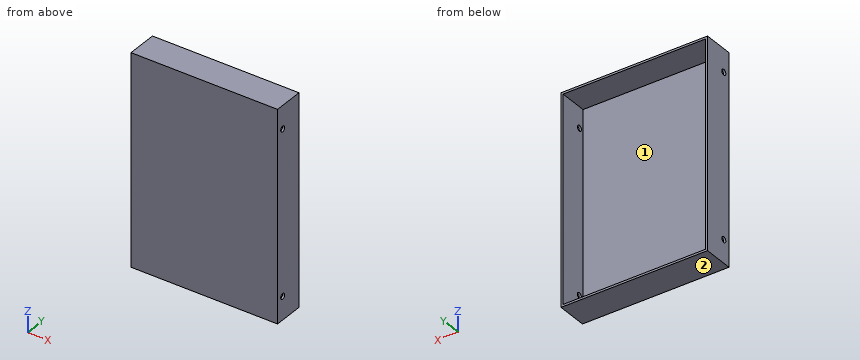
```python
from build123d import *

# Parameters (mm, degrees)
SKETCH1_W               = 350
SKETCH1_H               = 500
BOSS_EXTRUDE1_DEPTH     = 72.5
SHELL1_T                = -5
CUT_EXTRUDE1_DEPTH      = 437.183734222
CUT_EXTRUDE1_DEPTH_BACK = 437.183734222
SKETCH2_R               = 6.723131081


with BuildPart() as part:
    # Sketch1 → Boss-Extrude1 (new body)
    with BuildSketch(Plane(origin=(0, 0, 0), x_dir=(1, 0, 0), z_dir=(0, 1, 0))):
        Rectangle(SKETCH1_W, SKETCH1_H)
    extrude(amount=BOSS_EXTRUDE1_DEPTH)

    # Shell1
    shell1_openings = [part.faces().sort_by_distance(p)[0] for p in [
        (0, 72.5, 0),
    ]]
    offset(amount=SHELL1_T, openings=shell1_openings, kind=Kind.INTERSECTION)

    # Sketch2 → Cut-Extrude1 (cut, two sides: drawn at the far end of the back side and taken through both)
    with BuildSketch(Plane(origin=(175, 0, 0), x_dir=(0, 0, -1), z_dir=(1, 0, 0)).offset(-CUT_EXTRUDE1_DEPTH_BACK)):
        with Locations((-195, 17.5)):
            Circle(SKETCH2_R)
        with Locations((195, 17.5)):
            Circle(SKETCH2_R)
    extrude(amount=CUT_EXTRUDE1_DEPTH + CUT_EXTRUDE1_DEPTH_BACK, mode=Mode.SUBTRACT)


solid = part.part
```
Check sheet for the modelled part. Datum: model origin and axes. Units: mm. Face numbers are marked on the shaded views. A direction names the side the tool comes from. Coordinates: 2 decimals unless noted, no trailing zeros. Order: outer loops, then holes, each group sorted by start corner. A loop starts at its lowest first (then second) coordinate and runs counter-clockwise, first axis right, second up. Notation, with made-up numbers: M -40,48.5 L 8,48.5 A8 ccw 8,56.5 Z; hole C 80.25,-13.5 d6. An arc over 180 degrees is marked long. One line per question, with ' | ' between items. Start each with the question number.
Item 1: Gauge pin test, flat ends, axial feed: P1, Ø12, axis at y = 17.5, z = -195, coming from the +X side; P2, Ø6, axis at x = 70, z = 74.5, coming from the +Y side. Record the tip position at first contact, or that the pin passes through.
Item 2: Material ranges on line 1 (Z direction, x = -172.7, y = 17.5); line 2 (X direction, y = 33.5, z = -178); line 3 (Y direction, x = 171, z = -195), recorded low to high.
Item 3: Sectioned sample at B-B on y = 17.5. Record the cut outline in (x, z), and give its area (3 significant figures).
Item 4: Sectioned sample at D-D on y = 61. Record the cut outline in (x, z).
Item 5: Sectioned sample at C-C on x = -9.5. Record the cut outline in (y, z), and give its area (4 significant figures).
Item 6: Sectioned sample at A-A on z = -195. Record the cut outline in (x, y), and give its area (3 significant figures).
Item 7: Access from +Z, -Z, +X, -X, +Y, -Y to the whole of each face (thin tool, end or side, straight path). Record for the marked faces 1 and 2.
Answer below:
1) P1: passes through | P2: stops at y = 5
2) line 1: z = -250 to -201.72, -188.28 to 188.28, 201.72 to 250 | line 2: x = -175 to -170, 170 to 175 | line 3: y = 0 to 10.78, 24.22 to 72.5
3) outline: M -175,-250 L 175,-250 L 175,-201.72 L 170,-201.72 L 170,-245 L -170,-245 L -170,-201.72 L -175,-201.72 Z; M -175,-188.28 L -170,-188.28 L -170,188.28 L -175,188.28 Z; M -175,201.72 L -170,201.72 L -170,245 L 170,245 L 170,201.72 L 175,201.72 L 175,250 L -175,250 Z; M 170,-188.28 L 175,-188.28 L 175,188.28 L 170,188.28 Z | area: 8,130 mm^2
4) outline: M -175,-250 L 175,-250 L 175,250 L -175,250 Z; hole M -170,-245 L 170,-245 L 170,245 L -170,245 Z
5) outline: M 0,-250 L 72.5,-250 L 72.5,-245 L 5,-245 L 5,245 L 72.5,245 L 72.5,250 L 0,250 Z | area: 3,175 mm^2
6) outline: M -175,0 L 175,0 L 175,10.78 L 170,10.78 L 170,5 L -170,5 L -170,10.78 L -175,10.78 Z; M -175,24.22 L -170,24.22 L -170,72.5 L -175,72.5 Z; M 170,24.22 L 175,24.22 L 175,72.5 L 170,72.5 Z | area: 2,290 mm^2
7) face 1: +Y | face 2: -Z, +X, -X, +Y, -Y
